The listing builds one solid part. Answer for the finished solid, in the listing's coordinates (mm). Face numbers are marked on the shaded views. A direction names the side the tool comes from. Round coordinates to 2 decimals unless told otherwise and drop trailing zeros. Write each loop counter-clockwise with the first axis right and the second up, starting at its lowest first coordinate (ties: lowest second). Pieces come first, ordered by that corner, then holes. Notation, with made-up numbers: (71.5, 53.5) - (113.5, 53.5) arc R27 cw to (113.5, 78.5) - close; hole circle Ø5 at (74.5, 73). An arc over 180 degrees is marked (long way). Answer in a Markdown table with one row per item.
from build123d import *

# Parameters (mm, degrees)
SKETCH1_W           = 95.44
SKETCH1_H           = 80.2
SKETCH1_W_2         = 91.44
SKETCH1_H_2         = 76.2
BOSS_EXTRUDE1_DEPTH = 52.832
SKETCH2_W           = 139.7
SKETCH2_H           = 80.2
SKETCH2_R           = 3.15
BOSS_EXTRUDE2_DEPTH = 3
SKETCH3_R           = 5.35
CUT_EXTRUDE1_DEPTH  = 1
SKETCH4_R           = 3.3274
SKETCH4_R_2         = 1.3589
BOSS_EXTRUDE3_DEPTH = 12.7
CUT_EXTRUDE2_REACH  = 82.2
SKETCH5_W           = 55.88
SKETCH5_H           = 17.78
CUT_EXTRUDE3_REACH  = 82.2
SKETCH6_W           = 13
SKETCH6_H           = 19.8


with BuildPart() as part:
    # Sketch1 → Boss-Extrude1 (new body)
    with BuildSketch(Plane(origin=(0, 0, 0), x_dir=(1, 0, 0), z_dir=(0, 1, 0))):
        with Locations((2.309383501, -12.95659189)):
            Rectangle(SKETCH1_W, SKETCH1_H)
        with Locations((2.309383501, -12.95659189)):
            Rectangle(SKETCH1_W_2, SKETCH1_H_2, mode=Mode.SUBTRACT)
    extrude(amount=BOSS_EXTRUDE1_DEPTH)

    # Sketch2 → Boss-Extrude2 (add)
    with BuildSketch(Plane(origin=(0, 0, 0), x_dir=(1, 0, 0), z_dir=(0, 1, 0))):
        with Locations((2.309383501, -12.95659189)):
            Rectangle(SKETCH2_W, SKETCH2_H)
        with Locations((-60.190616499, 12.04340811)):
            Circle(SKETCH2_R, mode=Mode.SUBTRACT)
        with Locations((64.809383501, 12.04340811)):
            Circle(SKETCH2_R, mode=Mode.SUBTRACT)
        with Locations((-60.190616499, -37.95659189)):
            Circle(SKETCH2_R, mode=Mode.SUBTRACT)
        with Locations((64.809383501, -37.95659189)):
            Circle(SKETCH2_R, mode=Mode.SUBTRACT)
        with Locations((-60.190616499, -12.95659189)):
            Circle(SKETCH2_R, mode=Mode.SUBTRACT)
        with Locations((64.809383501, -12.95659189)):
            Circle(SKETCH2_R, mode=Mode.SUBTRACT)
    extrude(amount=BOSS_EXTRUDE2_DEPTH)

    # Sketch3 → Cut-Extrude1 (cut)
    with BuildSketch(Plane(origin=(0, 3, 0), x_dir=(1, 0, 0), z_dir=(0, 1, 0))):
        with Locations((-60.190616499, 12.04340811)):
            Circle(SKETCH3_R)
        with Locations((-60.190616499, -12.95659189)):
            Circle(SKETCH3_R)
        with Locations((-60.190616499, -37.95659189)):
            Circle(SKETCH3_R)
        with Locations((64.809383501, 12.04340811)):
            Circle(SKETCH3_R)
        with Locations((64.809383501, -12.95659189)):
            Circle(SKETCH3_R)
        with Locations((64.809383501, -37.95659189)):
            Circle(SKETCH3_R)
    extrude(amount=-CUT_EXTRUDE1_DEPTH, mode=Mode.SUBTRACT)

    # Sketch4 → Boss-Extrude3 (add)
    with BuildSketch(Plane(origin=(0, 3, 0), x_dir=(1, 0, 0), z_dir=(0, 1, 0))):
        with Locations((-28.170616499, 19.27600811)):
            Circle(SKETCH4_R)
        with Locations((-28.170616499, 19.27600811)):
            Circle(SKETCH4_R_2, mode=Mode.SUBTRACT)
        with Locations((32.789383501, 19.27600811)):
            Circle(SKETCH4_R)
        with Locations((32.789383501, 19.27600811)):
            Circle(SKETCH4_R_2, mode=Mode.SUBTRACT)
        with Locations((32.789383501, -16.28399189)):
            Circle(SKETCH4_R)
        with Locations((32.789383501, -16.28399189)):
            Circle(SKETCH4_R_2, mode=Mode.SUBTRACT)
        with Locations((-28.170616499, -16.28399189)):
            Circle(SKETCH4_R)
        with Locations((-28.170616499, -16.28399189)):
            Circle(SKETCH4_R_2, mode=Mode.SUBTRACT)
    extrude(amount=BOSS_EXTRUDE3_DEPTH)

    # Sketch5 → Cut-Extrude2 (cut, up to next)
    with BuildSketch(Plane(origin=(0, 0, -27.14340811), x_dir=(-1, 0, 0), z_dir=(0, 0, -1)), mode=Mode.PRIVATE) as cut_extrude2_sk1:
        with Locations((-2.309383501, 24.59)):
            Rectangle(SKETCH5_W, SKETCH5_H)
    cut_extrude2_tool1 = extrude(cut_extrude2_sk1.sketch, amount=-CUT_EXTRUDE2_REACH, mode=Mode.PRIVATE) & part.part
    add(cut_extrude2_tool1.solids().sort_by_distance((2.309384, 24.59, -27.143408))[0], mode=Mode.SUBTRACT)

    # Sketch6 → Cut-Extrude3 (cut, up to next)
    with BuildSketch(Plane.XY.offset(53.05659189), mode=Mode.PRIVATE) as cut_extrude3_sk1:
        with BuildLine():
            Line((-34.353116499, 40.137590136), (-34.353116499, 34.744409864))
            ThreePointArc((-34.353116499, 34.744409864), (-31.178116499, 33.2754), (-28.003116499, 34.744409864))
            Line((-28.003116499, 34.744409864), (-28.003116499, 40.137590136))
            ThreePointArc((-28.003116499, 40.137590136), (-31.178116499, 41.6066), (-34.353116499, 40.137590136))
        make_face()
    cut_extrude3_tool1 = extrude(cut_extrude3_sk1.sketch, amount=-CUT_EXTRUDE3_REACH, mode=Mode.PRIVATE) & part.part
    add(cut_extrude3_tool1.solids().sort_by_distance((-31.178116, 37.441, 53.056592))[0], mode=Mode.SUBTRACT)
    # Sketch6 → Cut-Extrude3 (cut, up to next)
    with BuildSketch(Plane.XY.offset(53.05659189), mode=Mode.PRIVATE) as cut_extrude3_sk2:
        with BuildLine():
            Line((-15.303116499, 40.137590136), (-15.303116499, 34.744409864))
            ThreePointArc((-15.303116499, 34.744409864), (-12.128116499, 33.2754), (-8.953116499, 34.744409864))
            Line((-8.953116499, 34.744409864), (-8.953116499, 40.137590136))
            ThreePointArc((-8.953116499, 40.137590136), (-12.128116499, 41.6066), (-15.303116499, 40.137590136))
        make_face()
    cut_extrude3_tool2 = extrude(cut_extrude3_sk2.sketch, amount=-CUT_EXTRUDE3_REACH, mode=Mode.PRIVATE) & part.part
    add(cut_extrude3_tool2.solids().sort_by_distance((-12.128116, 37.441, 53.056592))[0], mode=Mode.SUBTRACT)
    # Sketch6 → Cut-Extrude3 (cut, up to next)
    with BuildSketch(Plane.XY.offset(53.05659189), mode=Mode.PRIVATE) as cut_extrude3_sk3:
        with BuildLine():
            Line((3.746883501, 40.137590136), (3.746883501, 34.744409864))
            ThreePointArc((3.746883501, 34.744409864), (6.921883501, 33.2754), (10.096883501, 34.744409864))
            Line((10.096883501, 34.744409864), (10.096883501, 40.137590136))
            ThreePointArc((10.096883501, 40.137590136), (6.921883501, 41.6066), (3.746883501, 40.137590136))
        make_face()
    cut_extrude3_tool3 = extrude(cut_extrude3_sk3.sketch, amount=-CUT_EXTRUDE3_REACH, mode=Mode.PRIVATE) & part.part
    add(cut_extrude3_tool3.solids().sort_by_distance((6.921884, 37.441, 53.056592))[0], mode=Mode.SUBTRACT)
    # Sketch6 → Cut-Extrude3 (cut, up to next)
    with BuildSketch(Plane.XY.offset(53.05659189), mode=Mode.PRIVATE) as cut_extrude3_sk4:
        with BuildLine():
            Line((-34.353116499, 21.087590136), (-34.353116499, 15.694409864))
            ThreePointArc((-34.353116499, 15.694409864), (-31.178116499, 14.2254), (-28.003116499, 15.694409864))
            Line((-28.003116499, 15.694409864), (-28.003116499, 21.087590136))
            ThreePointArc((-28.003116499, 21.087590136), (-31.178116499, 22.5566), (-34.353116499, 21.087590136))
        make_face()
    cut_extrude3_tool4 = extrude(cut_extrude3_sk4.sketch, amount=-CUT_EXTRUDE3_REACH, mode=Mode.PRIVATE) & part.part
    add(cut_extrude3_tool4.solids().sort_by_distance((-31.178116, 18.391, 53.056592))[0], mode=Mode.SUBTRACT)
    # Sketch6 → Cut-Extrude3 (cut, up to next)
    with BuildSketch(Plane.XY.offset(53.05659189), mode=Mode.PRIVATE) as cut_extrude3_sk5:
        with BuildLine():
            Line((3.746883501, 21.087590136), (3.746883501, 15.694409864))
            ThreePointArc((3.746883501, 15.694409864), (6.921883501, 14.2254), (10.096883501, 15.694409864))
            Line((10.096883501, 15.694409864), (10.096883501, 21.087590136))
            ThreePointArc((10.096883501, 21.087590136), (6.921883501, 22.5566), (3.746883501, 21.087590136))
        make_face()
    cut_extrude3_tool5 = extrude(cut_extrude3_sk5.sketch, amount=-CUT_EXTRUDE3_REACH, mode=Mode.PRIVATE) & part.part
    add(cut_extrude3_tool5.solids().sort_by_distance((6.921884, 18.391, 53.056592))[0], mode=Mode.SUBTRACT)
    # Sketch6 → Cut-Extrude3 (cut, up to next)
    with BuildSketch(Plane.XY.offset(53.05659189), mode=Mode.PRIVATE) as cut_extrude3_sk6:
        with Locations((32.471883501, 27.916)):
            Rectangle(SKETCH6_W, SKETCH6_H)
    cut_extrude3_tool6 = extrude(cut_extrude3_sk6.sketch, amount=-CUT_EXTRUDE3_REACH, mode=Mode.PRIVATE) & part.part
    add(cut_extrude3_tool6.solids().sort_by_distance((32.471884, 27.916, 53.056592))[0], mode=Mode.SUBTRACT)


solid = part.part
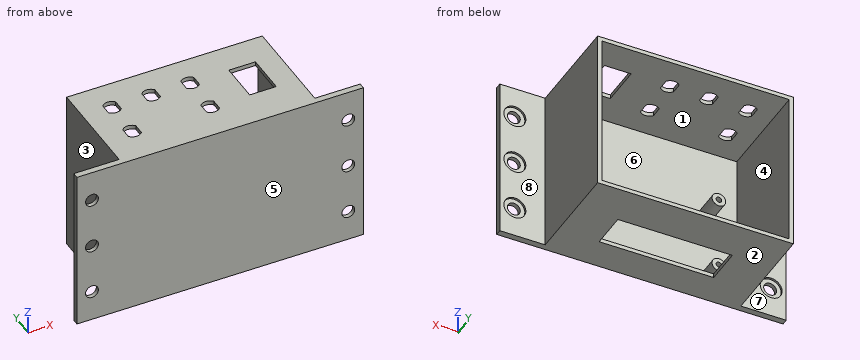
(1) Section D-D (z = 21.5) is taken. Give the vertices of the cut face in (x, y).
Checked values:
| item | result |
|---|---|
| outline | (-67.54, 0) - (72.16, 0) - (72.16, 3) - (50.03, 3) - (50.03, 52.83) - (48.03, 52.83) - (48.03, 3) - (-43.41, 3) - (-43.41, 52.83) - (-45.41, 52.83) - (-45.41, 3) - (-67.54, 3) - close |
(2) Section A-A (y = 24.5) is taken. Give the vertices of the cut face in (x, z), and give its area (3 significant figures).
Checked values:
| item | result |
|---|---|
| outline | (-45.41, -27.14) - (-25.63, -27.14) - (-25.63, -25.14) - (-43.41, -25.14) - (-43.41, 51.06) - (25.97, 51.06) - (25.97, 53.06) - (-45.41, 53.06) - close; (30.25, -27.14) - (50.03, -27.14) - (50.03, 53.06) - (38.97, 53.06) - (38.97, 51.06) - (48.03, 51.06) - (48.03, -25.14) - (30.25, -25.14) - close |
| area | 549 mm2 |
(3) Section B-B (x = 21.5) is taken. Give the vertices of the cut face in (y, z), and give its area (3 significant figures).
Checked values:
| item | result |
|---|---|
| outline | (0, -27.14) - (15.7, -27.14) - (15.7, -25.14) - (3, -25.14) - (3, 51.06) - (52.83, 51.06) - (52.83, 53.06) - (0, 53.06) - close; (33.48, -27.14) - (52.83, -27.14) - (52.83, -25.14) - (33.48, -25.14) - close |
| area | 404 mm2 |
(4) For a pull along X with two mould halves and no side action, classify the marked faces 1, 2, 3 and 4 as pulls with the +X half, pulls with the -X half, needs draft (parallel to the pull), parting line crosses it, or undercut.
Checked values:
| item | result |
|---|---|
| face 1 | undercut |
| face 2 | needs draft |
| face 3 | pulls with the -X half |
| face 4 | undercut |
(5) Flat-ended cylindrical pins translate along their axes: pin 1 (4.5 mm diameter, centred on x = -28.17, z = -19.28, fed in from +Y); pin 2 (2 mm diameter, centred on x = -21.5, z = -14, fed in from +Y); pin 3 (1 mm diameter, centred on y = 25, z = -26, fed in from -X); pin 4 (4 mm diameter, centred on x = 37, z = 40, fed in from -Y). Find the tip coordinate at first contact, or state that the pin passes through.
Checked values:
| item | result |
|---|---|
| pin 1 | stops at y = 15.7 |
| pin 2 | stops at y = 3 |
| pin 3 | stops at x = -45.41 |
| pin 4 | stops at y = 0 |
(6) Section C-C (y = 7.5) is taken. State how many separate pieces and enclosed holes the cut face has, and give its area (3 significant figures).
Checked values:
| item | result |
|---|---|
| separate pieces | 5 |
| enclosed holes | 5 |
| area | 802 mm2 |
(7) For the marked faces 5, 6, 7 and 8, determine the directions among +Z, -Z, +X, -X, +Y, -Y from which every point of the face is accessible in a straight line to the end or side of a thin tool.
Checked values:
| item | result |
|---|---|
| face 5 | +Z, -Z, +X, -X, -Y |
| face 6 | +Y |
| face 7 | +Z, -Z, -X, +Y |
| face 8 | +Z, -Z, +X, +Y |
(8) Find the intervals of material crossed by line 1 (Z direction, x = -7, y = 5); line 2 (X direction, y = 21, z = 34); line 3 (Y direction, x = 46, z = -16), in increasing order.
Checked values:
| item | result |
|---|---|
| line 1 | z = -27.14 to -25.14, 51.06 to 53.06 |
| line 2 | x = -45.41 to -43.41, 48.03 to 50.03 |
| line 3 | y = 0 to 3 |
